Autodesk Fusion 360 part; units mm, degrees
sketch "Sketch2" plane through (0, 0, 0) normal (1, 0, 0) x (0, 0, -1)
  line L0 (0, 0) -> (30, 70)
  line L1 (30, 70) -> (90, 70)
  line L2 (90, 70) -> (150, 0)
  line L3 (150, 0) -> (0, 0)
  line L4 (36.594, 60) -> (85.4007, 60)
  line L5 (85.4007, 60) -> (128.2578, 10)
  line L6 (128.2578, 10) -> (15.1654, 10)
  line L7 (15.1654, 10) -> (36.594, 60)
  dimension "d9" = 10
  dimension "d10" = 70
  dimension "d11" = 30
  dimension "d12" = 60
  dimension "d13" = 60
extrude "Extrude1" add sketch "Sketch2" along normal blind 100
sketch "Sketch3" plane through (0, 70, 0) normal (0, 1, 0) x (-1, 0, 0)
  line L0 (0, -90) -> (0, -30)
  line L1 (0, -30) -> (-100, -30)
  line L2 (-100, -30) -> (-100, -90)
  line L3 (-100, -90) -> (0, -90)
  line L4 (-100, -30) -> (0, -30) construction
  line L5 (-50, -30) -> (-50, -100) construction
  line L6 (-20, -150) -> (-80, -150)
  line L7 (-80, -150) -> (-80, -50)
  line L8 (-80, -50) -> (-20, -50)
  line L9 (-20, -50) -> (-20, -150)
  line L10 (-20, -150) -> (-80, -50) construction
  line L11 (-80, -150) -> (-20, -50) construction
  point P0 (-50, -100)
  dimension "d19" = 70
  dimension "d20" = 60
  dimension "d21" = 100
extrude "Extrude2" cut sketch "Sketch3" along normal through all contours L3 L6 L7 L9 | L3 L7 L8 L9
Can you work these out from the model? Positions are in its coordinate system, mm. A direction names the side the tool comes from. Round coordinates to 2 decimals unless told otherwise and drop trailing zeros. Loops run counter-clockwise (first coordinate to the right, second up) from the corner with the lowest first, then second, coordinate; pieces in that order, holes last.
Item 1: Will these pins go through, and if not, where does the flat tip stop? pin 1 Ø1 at (x, y) = (15.5, 38) entering from +Z; pin 2 Ø4 at (x, y) = (72.5, 22) entering from -Z; pin 3 Ø4 at (x, y) = (77, 28) entering from +Z.
Item 2: Suppose I cut it at C-C, the plane y = 44.5. Write out the boundary of the cut face in (x, z), then the cut area to 3 significant figures.
Item 3: Suppose I cut it at A-A, the plane x = 10. Write out the boundary of the cut face in (y, z), then the cut area to 3 significant figures.
Item 4: Please list where these lines run through material, in increasing order: L1, parallel to Z at x = 86, y = 16; L2, parallel to Z at x = 71.5, y = 22; L3, parallel to Y at x = 23.5, z = -96.
Item 5: If we mould it in two halves opening along Z, with no side actions, what happens to faces 1 (the flat face through (49, 0, -76)), 2 (the flat face through (49, 35, -120)), 3 (the flat face through (49, 10, -73))? For each: +Z half, -Z half, draft (parallel to the pull), parting line (faces both ways), or undercut.
Item 6: Suppose I cut it at D-D, the plane z = -139.5. Write out the boundary of the cut face in (x, y), then the cut area to 4 significant figures.
Item 7: Which directions (+Z, -Z, +X, -X, +Y, -Y) give clear straight access to the entire face, cutting with the end or side of a thin tool? Please do faces 4 (the flat face through (49, 60, -61)), 5 (the flat face through (100, 9, -69)).
Item 8: Suppose I cut it at B-B, the plane z = -70. Write out the boundary of the cut face in (x, y).
Reported:
1. pin 1: stops at z = -16.07
1. pin 2: stops at z = -132.86
1. pin 3: stops at z = -11.14
2. outline: (0, -111.86) - (100, -111.86) - (100, -98.69) - (0, -98.69) - close; (0, -29.95) - (100, -29.95) - (100, -19.07) - (0, -19.07) - close
2. area: 2,410 mm2
3. outline: (0, -150) - (70, -90) - (70, -30) - (0, 0) - close; hole (10, -128.26) - (60, -85.4) - (60, -36.59) - (10, -15.17) - close
3. area: 3,300 mm2
4. L1: z = -136.29 to -123.11, -17.74 to -6.86
4. L2: z = -131.14 to -117.97, -20.31 to -9.43
4. L3: y = 0 to 10, 47.63 to 63
5. face 1: draft
5. face 2: -Z half
5. face 3: undercut
6. outline: (0, 0) - (100, 0) - (100, 12.25) - (0, 12.25) - close
6. area: 1,225 mm2
7. face 4: +X, -X
7. face 5: +Z, -Z, +X, +Y, -Y
8. outline: (0, 0) - (100, 0) - (100, 10) - (0, 10) - close; (0, 60) - (100, 60) - (100, 70) - (0, 70) - close
